Work out the finished part from the listing and answer in its coordinate system (mm). A direction names the side the tool comes from. Give positions to 0.01 mm unless a question says otherwise; leave off trailing zeros. Order: outer loops, then holes, each group sorted by start corner. A loop starts at its lowest first (then second) coordinate and runs counter-clockwise, first axis right, second up. Notation, with made-up numbers: M -6.5,63 L 34.5,63 A19 ccw 34.5,96 Z; hole C 3.25,12.5 d2. An arc over 180 degrees is marked long. One line per item, written item: value.
Autodesk Fusion 360 part; units mm, degrees
sketch "Skizze1" plane through (0, 0, 0) normal (0, 0, 1) x (1, 0, 0)
  line L0 (0, 0) -> (60, 0)
  line L1 (60, 0) -> (60, 20)
  line L2 (60, 20) -> (0, 20)
  line L3 (0, 20) -> (0, 0)
  circle A0 centre (53.2, 5.4) radius 1.275
  circle A1 centre (53.2, 15.1) radius 1.275
  line L4 (0, 20) -> (30, 20)
  line L5 (30, 20) -> (30, 0)
  line L6 (30, 0) -> (0, 0)
  line L7 (0, 0) -> (0, 20)
  dimension "d1" = 60
  dimension "d2" = 20
  dimension "d3" = 2.55
  dimension "d4" = 2.55
  dimension "d5" = 5.4
  dimension "d6" = 6.8
  dimension "d7" = 4.9
  dimension "d8" = 6.8
extrude "Extrusion1" add sketch "Skizze1" along normal blind 6
extrude "Extrusion2" add sketch "Skizze1" along normal blind 14 contours A0 | A1
extrude "Extrusion3" add sketch "Skizze1" against normal blind 5 contours L0 L2 L3 L4 L5 L6 L7
sketch "Skizze2" plane through (0, 0, 0) normal (0, -1, 0) x (1, 0, 0)
  line L0 (30, 0) -> (60, 0)
  line L1 (60, 0) -> (60, 6)
  line L2 (60, 6) -> (0, 6)
  line L3 (0, 6) -> (0, -5)
  line L4 (0, -5) -> (30, -5)
  line L5 (30, -5) -> (30, 0)
  line L6 (30, -5) -> (60, 0)
  line L7 (0, 6) -> (30, 6)
  line L8 (30, 6) -> (30, 0)
  line L9 (30, 0) -> (0, 0)
  line L10 (0, 0) -> (0, 6)
  line L11 (30, 6) -> (24.9654, 0)
  line L12 (30, 6) -> (37.8324, 6) construction
  line L13 (0, -5) -> (30, -5)
  line L14 (30, -5) -> (30, -10)
  line L15 (30, -10) -> (0, -10)
  line L16 (0, -10) -> (0, -5)
  dimension "d41" = 130
  dimension "d44" = 5
extrude "Extrusion6" add sketch "Skizze2" against normal blind 20 contours L0 L5 L6
extrude "Extrusion7" cut sketch "Skizze2" against normal blind 20 contours L2 L3 L7 L9 L10 L11
extrude "Extrusion8" add sketch "Skizze2" against normal blind 20 contours L4 L13 L14 L15 L16
hole "Bohrung5" at (5.0685, 15.1186, 0) direction (0, 0, -1) diameter 3.5 depth 10 tip angle 180 countersink diameter 5.5 countersink angle 90
hole "Bohrung6" at (19.9516, 5.0738, 0) direction (0, 0, -1) diameter 3.5 depth 10 tip angle 180 countersink diameter 5.5 countersink angle 90
equation "d6 = 5.7 mm + 1.1 mm"
equation "d8 = 5.7 mm + 1.1 mm"
(1) Given P1, Ø6, axis at x = 41, y = 11.5, coming from the +Z side; P2, Ø1.5, axis at y = 11.5, z = -6.5, coming from the +X side; P3, Ø2, axis at x = 9, y = 17, coming from the +Z side, each flat-ended and moving along its own axis, determine where each tip first touches the part or whether it passes through.
Findings:
P1: stops at z = 6
P2: stops at x = 30
P3: stops at z = 0
(2) Section B-B, the plane x = 53.2 is taken. Give the vertices of the cut face in (y, z) (3 decimals), then the cut area to 3 significant figures.
Findings:
outline: M 0,-1.133 L 20,-1.133 L 20,6 L 16.375,6 L 16.375,14 L 13.825,14 L 13.825,6 L 6.675,6 L 6.675,14 L 4.125,14 L 4.125,6 L 0,6 Z
area: 183 mm^2
(3) Section D-D, the plane x = 42 is taken. Give the vertices of the cut face in (y, z), then the cut area to 3 significant figures.
Findings:
outline: M 0,-3 L 20,-3 L 20,6 L 0,6 Z
area: 180 mm^2
(4) Find the intervals of material crossed by probe 1 along Z at (x, y) = (9, 10.5); probe 2 along Z at (x, y) = (33, 9.75); probe 3 along X at (y, z) = (4, -5.75), in increasing order. Write a range as from..to.
Findings:
probe 1: z = -10..0
probe 2: z = -4.5..6
probe 3: x = 0..18.57, 21.33..30
(5) Determine the mould class of faces 1 (the cylindrical face through (21.504, 4.266, -5.563)), 2 (the flat face through (53, 15, 14)), 3 (the flat face through (30, 0, -2)) for opening direction Y: pulls with the +Y half, pulls with the -Y half, needs draft (parallel to the pull), parting line crosses it, or undercut.
Findings:
face 1: undercut
face 2: needs draft
face 3: pulls with the -Y half
(6) Which of the six approach directions +Z, -Z, +X, -X, +Y, -Y give full straight-line access (tool end or side, diameter ignored) to faces 4 (the cylindrical face through (3.89, 16.41, -5.56)), 5 (the flat face through (13, 10, 0)), 6 (the flat face through (30, 10, -7)), 7 (the cylindrical face through (52.26, 14.24, 9.94)), 8 (the flat face through (60, 10, 3))?
Findings:
face 4: +Z, -Z
face 5: +Z, -X, +Y, -Y
face 6: -Z, +X, +Y, -Y
face 7: +Z
face 8: +Z, -Z, +X, +Y, -Y
(7) Section C-C, the plane z = 1 is taken. Give the vertices of the cut face in (x, y).
Findings:
outline: M 25.8,0 L 60,0 L 60,20 L 25.8,20 Z
(8) Section A-A, the plane y = 8.75 is taken. Give the vertices of the cut face in (x, z).
Findings:
outline: M 0,-10 L 30,-10 L 30,-5 L 60,0 L 60,6 L 30,6 L 24.97,0 L 0,0 Z
